The listing builds one solid part. Answer for the finished solid, in the listing's coordinates (mm). Give positions to 0.01 mm unless a question says otherwise; leave off trailing zeros. Loops run counter-clockwise (first coordinate to the right, second up) from the corner with the lowest first, then second, coordinate; pieces in that order, holes last.
Item 1: Section C-C, the plane y = -23 is taken. Give the vertices of the cut face in (x, z), and give its area (3 significant figures).
Item 2: Section B-B, the plane x = -7.5 is taken. Give the vertices of the cut face in (y, z), and give its area (3 significant figures).
Item 3: Consider line 1 along Y through (x, z) = (-45.75, 1.5); line 2 along Y through (x, z) = (11.5, 2.5); line 3 along Y through (x, z) = (-26, 7). Determine where each line is inside the solid, lowest interval first.
Item 4: Section A-A, the plane y = 45 is taken. Give the vertices of the cut face in (x, z), and give its area (4 significant figures).
Item 5: Each of these flat-tipped pins is pushed along its axis until it touches: pin 1 Ø2.5 at (x, z) = (0.5, 5.5) entering from +Y; pin 2 Ø3 at (x, y) = (38.5, -34.5) entering from +Z; pin 3 Ø4.5 at (x, z) = (-13, 5) entering from -Y. Where does it stop, or does it pass through?
from build123d import *

# Parameters (mm, degrees)
SKETCH1_W           = 100
SKETCH1_H           = 113.5
BOSS_EXTRUDE1_DEPTH = 8.5
CUT_EXTRUDE1_REACH  = 78.111
SKETCH2_W           = 83
SKETCH2_H           = 13.5
SKETCH2_H_2         = 13
SKETCH2_W_2         = 10
SKETCH2_H_3         = 10
SKETCH2_R           = 1.75
CUT_EXTRUDE2_REACH  = 78.111
SKETCH6_W           = 10
SKETCH6_H           = 10
FILLET1_R           = 1
SKETCH8_W           = 10
SKETCH8_H           = 10
CUT_EXTRUDE5_DEPTH  = 5.5
CUT_EXTRUDE6_DEPTH  = 76.834111718


with BuildPart() as part:
    # Sketch1 → Boss-Extrude1 (new body)
    with BuildSketch(Plane.XY):
        Rectangle(SKETCH1_W, SKETCH1_H)
    extrude(amount=BOSS_EXTRUDE1_DEPTH)

    # Sketch2 → Cut-Extrude1 (cut, up to next)
    with BuildSketch(Plane.XY.offset(8.5), mode=Mode.PRIVATE) as cut_extrude1_sk1:
        with Locations((0, 50)):
            Rectangle(SKETCH2_W, SKETCH2_H)
    cut_extrude1_tool1 = extrude(cut_extrude1_sk1.sketch, amount=-CUT_EXTRUDE1_REACH, mode=Mode.PRIVATE) & part.part
    # Sketch2 → Cut-Extrude1 (cut, up to next)
    with BuildSketch(Plane.XY.offset(8.5), mode=Mode.PRIVATE) as cut_extrude1_sk2:
        with BuildLine():
            ThreePointArc((-41.5, -29.75), (-39.156854249, -35.406854249), (-33.5, -37.75))
            Line((-33.5, -37.75), (33.5, -37.75))
            ThreePointArc((33.5, -37.75), (39.156854249, -35.406854249), (41.5, -29.75))
            Line((41.5, -29.75), (41.5, -0.25))
            Line((41.5, -0.25), (-41.5, -0.25))
            Line((-41.5, -0.25), (-41.5, -29.75))
        make_face()
    cut_extrude1_tool2 = extrude(cut_extrude1_sk2.sketch, amount=-CUT_EXTRUDE1_REACH, mode=Mode.PRIVATE) & part.part
    # Sketch2 → Cut-Extrude1 (cut, up to next)
    with BuildSketch(Plane.XY.offset(8.5), mode=Mode.PRIVATE) as cut_extrude1_sk3:
        with Locations((0, -50.25)):
            Rectangle(SKETCH2_W, SKETCH2_H_2)
    cut_extrude1_tool3 = extrude(cut_extrude1_sk3.sketch, amount=-CUT_EXTRUDE1_REACH, mode=Mode.PRIVATE) & part.part
    # Sketch2 → Cut-Extrude1 (cut, up to next)
    with BuildSketch(Plane.XY.offset(8.5), mode=Mode.PRIVATE) as cut_extrude1_sk4:
        with Locations((-11.75, 22.75)):
            Rectangle(SKETCH2_W_2, SKETCH2_H_3)
    cut_extrude1_tool4 = extrude(cut_extrude1_sk4.sketch, amount=-CUT_EXTRUDE1_REACH, mode=Mode.PRIVATE) & part.part
    # Sketch2 → Cut-Extrude1 (cut, up to next)
    with BuildSketch(Plane.XY.offset(8.5), mode=Mode.PRIVATE) as cut_extrude1_sk5:
        with Locations((45.75, 38.75)):
            Circle(SKETCH2_R)
    cut_extrude1_tool5 = extrude(cut_extrude1_sk5.sketch, amount=-CUT_EXTRUDE1_REACH, mode=Mode.PRIVATE) & part.part
    # Sketch2 → Cut-Extrude1 (cut, up to next)
    with BuildSketch(Plane.XY.offset(8.5), mode=Mode.PRIVATE) as cut_extrude1_sk6:
        with Locations((45.75, -38.75)):
            Circle(SKETCH2_R)
    cut_extrude1_tool6 = extrude(cut_extrude1_sk6.sketch, amount=-CUT_EXTRUDE1_REACH, mode=Mode.PRIVATE) & part.part
    # Sketch2 → Cut-Extrude1 (cut, up to next)
    with BuildSketch(Plane.XY.offset(8.5), mode=Mode.PRIVATE) as cut_extrude1_sk7:
        with Locations((-45.75, 38.75)):
            Circle(SKETCH2_R)
    cut_extrude1_tool7 = extrude(cut_extrude1_sk7.sketch, amount=-CUT_EXTRUDE1_REACH, mode=Mode.PRIVATE) & part.part
    # Sketch2 → Cut-Extrude1 (cut, up to next)
    with BuildSketch(Plane.XY.offset(8.5), mode=Mode.PRIVATE) as cut_extrude1_sk8:
        with Locations((-45.75, -38.75)):
            Circle(SKETCH2_R)
    cut_extrude1_tool8 = extrude(cut_extrude1_sk8.sketch, amount=-CUT_EXTRUDE1_REACH, mode=Mode.PRIVATE) & part.part
    add(cut_extrude1_tool1.solids().sort_by_distance((0, 50, 8.5))[0], mode=Mode.SUBTRACT)
    add(cut_extrude1_tool2.solids().sort_by_distance((0, -18.848961, 8.5))[0], mode=Mode.SUBTRACT)
    add(cut_extrude1_tool3.solids().sort_by_distance((0, -50.25, 8.5))[0], mode=Mode.SUBTRACT)
    add(cut_extrude1_tool4.solids().sort_by_distance((-11.75, 22.75, 8.5))[0], mode=Mode.SUBTRACT)
    add(cut_extrude1_tool5.solids().sort_by_distance((45.75, 38.75, 8.5))[0], mode=Mode.SUBTRACT)
    add(cut_extrude1_tool6.solids().sort_by_distance((45.75, -38.75, 8.5))[0], mode=Mode.SUBTRACT)
    add(cut_extrude1_tool7.solids().sort_by_distance((-45.75, 38.75, 8.5))[0], mode=Mode.SUBTRACT)
    add(cut_extrude1_tool8.solids().sort_by_distance((-45.75, -38.75, 8.5))[0], mode=Mode.SUBTRACT)

    # Sketch6 → Cut-Extrude2 (cut, up to next)
    with BuildSketch(Plane.XY.offset(8.5), mode=Mode.PRIVATE) as cut_extrude2_sk1:
        with BuildLine():
            Line((41.5, 8.25), (41.5, 29.25))
            ThreePointArc((41.5, 29.25), (39.156854249, 34.906854249), (33.5, 37.25))
            Line((33.5, 37.25), (28.5, 37.25))
            Line((28.5, 37.25), (28.5, 8.25))
            Line((28.5, 8.25), (33.5, 8.25))
            Line((33.5, 8.25), (41.5, 8.25))
        make_face()
    cut_extrude2_tool1 = extrude(cut_extrude2_sk1.sketch, amount=-CUT_EXTRUDE2_REACH, mode=Mode.PRIVATE) & part.part
    # Sketch6 → Cut-Extrude2 (cut, up to next)
    with BuildSketch(Plane.XY.offset(8.5), mode=Mode.PRIVATE) as cut_extrude2_sk2:
        with Locations((11.75, 22.75)):
            Rectangle(SKETCH6_W, SKETCH6_H)
    cut_extrude2_tool2 = extrude(cut_extrude2_sk2.sketch, amount=-CUT_EXTRUDE2_REACH, mode=Mode.PRIVATE) & part.part
    # Sketch6 → Cut-Extrude2 (cut, up to next)
    with BuildSketch(Plane.XY.offset(8.5), mode=Mode.PRIVATE) as cut_extrude2_sk3:
        with BuildLine():
            Line((-41.5, 8.25), (-41.5, 29.25))
            ThreePointArc((-41.5, 29.25), (-39.156854249, 34.906854249), (-33.5, 37.25))
            Line((-33.5, 37.25), (-28.5, 37.25))
            Line((-28.5, 37.25), (-28.5, 8.25))
            Line((-28.5, 8.25), (-33.5, 8.25))
            Line((-33.5, 8.25), (-41.5, 8.25))
        make_face()
    cut_extrude2_tool3 = extrude(cut_extrude2_sk3.sketch, amount=-CUT_EXTRUDE2_REACH, mode=Mode.PRIVATE) & part.part
    add(cut_extrude2_tool1.solids().sort_by_distance((34.821806, 22.269339, 8.5))[0], mode=Mode.SUBTRACT)
    add(cut_extrude2_tool2.solids().sort_by_distance((11.75, 22.75, 8.5))[0], mode=Mode.SUBTRACT)
    add(cut_extrude2_tool3.solids().sort_by_distance((-34.821806, 22.269339, 8.5))[0], mode=Mode.SUBTRACT)

    # Fillet1
    fillet1_edges = [part.edges().sort_by_distance(p)[0] for p in [
        (45.75, -56.75, 0),
        (-45.75, 56.75, 0),
        (-45.75, -56.75, 8.5),
        (-45.75, 56.75, 8.5),
        (45.75, -56.75, 8.5),
        (-41.5, 56.75, 4.25),
        (41.5, 56.75, 4.25),
        (41.5, -56.75, 4.25),
        (-41.5, -56.75, 4.25),
        (-45.75, -56.75, 0),
        (45.75, 56.75, 0),
        (50, -56.75, 4.25),
        (-50, -56.75, 4.25),
        (-50, 56.75, 4.25),
        (50, 56.75, 4.25),
        (45.75, 56.75, 8.5),
    ]]
    fillet(fillet1_edges, radius=FILLET1_R)

    # Sketch8 → Cut-Extrude5 (cut)
    with BuildSketch(Plane.XY.offset(8.5)):
        with BuildLine():
            ThreePointArc((-46.701116722, 32.72), (-46.210984272, 34.031299083), (-44.981116722, 34.7))
            ThreePointArc((-44.981116722, 34.7), (-42.571113581, 35.629410248), (-40.811116722, 37.52))
            Line((-40.811116722, 37.52), (-39.567050808, 39.7))
            ThreePointArc((-39.567050808, 39.7), (-38.836346779, 40.434383498), (-37.835, 40.7))
            Line((-37.835, 40.7), (37.835, 40.7))
            ThreePointArc((37.835, 40.7), (38.836346779, 40.434383498), (39.567050808, 39.7))
            Line((39.567050808, 39.7), (40.811116722, 37.52))
            ThreePointArc((40.811116722, 37.52), (42.571113581, 35.629410248), (44.981116722, 34.7))
            ThreePointArc((44.981116722, 34.7), (46.210984272, 34.031299083), (46.701116722, 32.72))
            Line((46.701116722, 32.72), (46.701116722, -32.72))
            ThreePointArc((46.701116722, -32.72), (46.210984272, -34.031299083), (44.981116722, -34.7))
            ThreePointArc((44.981116722, -34.7), (42.571113581, -35.629410248), (40.811116722, -37.52))
            Line((40.811116722, -37.52), (39.567050808, -39.7))
            ThreePointArc((39.567050808, -39.7), (38.836346779, -40.434383498), (37.835, -40.7))
            Line((37.835, -40.7), (-37.835, -40.7))
            Line((-37.835, -40.7), (-39.567050808, -39.7))
            Line((-39.567050808, -39.7), (-40.811116722, -37.52))
            ThreePointArc((-40.811116722, -37.52), (-42.571113581, -35.629410248), (-44.981116722, -34.7))
            ThreePointArc((-44.981116722, -34.7), (-46.210984272, -34.031299083), (-46.701116722, -32.72))
            Line((-46.701116722, -32.72), (-46.701116722, 32.72))
        make_face()
        with Locations((-11.75, 22.75)):
            Rectangle(SKETCH8_W, SKETCH8_H, mode=Mode.SUBTRACT)
        with BuildLine():
            Line((33.5, -37.75), (-33.5, -37.75))
            ThreePointArc((-33.5, -37.75), (-39.156854249, -35.406854249), (-41.5, -29.75))
            Line((-41.5, -29.75), (-41.5, -0.25))
            Line((-41.5, -0.25), (41.5, -0.25))
            Line((41.5, -0.25), (41.5, -29.75))
            ThreePointArc((41.5, -29.75), (39.156854249, -35.406854249), (33.5, -37.75))
        make_face(mode=Mode.SUBTRACT)
        with Locations((11.75, 22.75)):
            Rectangle(SKETCH8_W, SKETCH8_H, mode=Mode.SUBTRACT)
        with BuildLine():
            Line((-41.5, 8.25), (-41.5, 29.25))
            ThreePointArc((-41.5, 29.25), (-39.156854249, 34.906854249), (-33.5, 37.25))
            Line((-33.5, 37.25), (-28.5, 37.25))
            Line((-28.5, 37.25), (-28.5, 8.25))
            Line((-28.5, 8.25), (-41.5, 8.25))
        make_face(mode=Mode.SUBTRACT)
        with BuildLine():
            Line((41.5, 8.25), (28.5, 8.25))
            Line((28.5, 8.25), (28.5, 37.25))
            Line((28.5, 37.25), (33.5, 37.25))
            ThreePointArc((33.5, 37.25), (39.156854249, 34.906854249), (41.5, 29.25))
            Line((41.5, 29.25), (41.5, 8.25))
        make_face(mode=Mode.SUBTRACT)
    extrude(amount=-CUT_EXTRUDE5_DEPTH, mode=Mode.SUBTRACT)

    # Sketch9 → Cut-Extrude6 (cut, through all)
    with BuildSketch(Plane.XY.offset(3)):
        with BuildLine():
            Line((-33.5, -37.75), (33.5, -37.75))
            ThreePointArc((33.5, -37.75), (39.156854249, -35.406854249), (41.5, -29.75))
            Line((41.5, -29.75), (41.5, 29.25))
            ThreePointArc((41.5, 29.25), (39.156854249, 34.906854249), (33.5, 37.25))
            Line((33.5, 37.25), (-33.5, 37.25))
            ThreePointArc((-33.5, 37.25), (-39.156854249, 34.906854249), (-41.5, 29.25))
            Line((-41.5, 29.25), (-41.5, -29.75))
            ThreePointArc((-41.5, -29.75), (-39.156854249, -35.406854249), (-33.5, -37.75))
        make_face()
    extrude(amount=-CUT_EXTRUDE6_DEPTH, mode=Mode.SUBTRACT)


solid = part.part
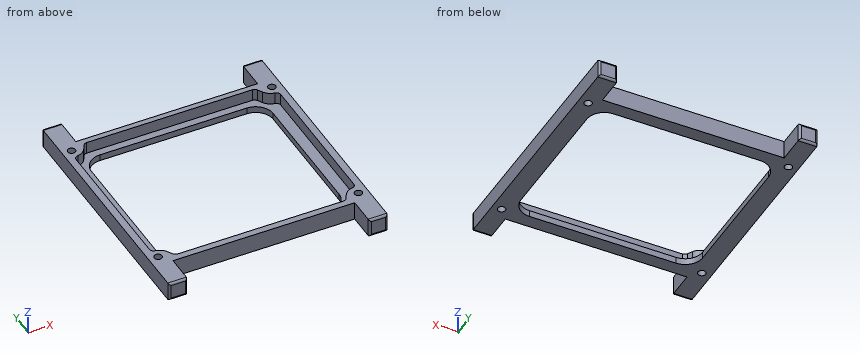
Worked answers:
1. outline: (-50, 0) - (-41.5, 0) - (-41.5, 3) - (-46.7, 3) - (-46.7, 8.5) - (-50, 8.5) - close; (41.5, 0) - (50, 0) - (50, 8.5) - (46.7, 8.5) - (46.7, 3) - (41.5, 3) - close
1. area: 87.3 mm2
2. outline: (-43.75, 0) - (-37.75, 0) - (-37.75, 3) - (-40.7, 3) - (-40.7, 8.5) - (-43.75, 8.5) - close; (37.25, 0) - (43.25, 0) - (43.25, 8.5) - (40.7, 8.5) - (40.7, 3) - (37.25, 3) - close
2. area: 66.8 mm2
3. line 1: y = -56.75 to -40.5, -37 to 37, 40.5 to 56.75
3. line 2: y = -43.75 to -37.75, 37.25 to 43.25
3. line 3: y = -43.75 to -40.7, 40.7 to 43.25
4. outline: (-50, 0) - (-41.5, 0) - (-41.5, 8.5) - (-50, 8.5) - close; (41.5, 0) - (50, 0) - (50, 8.5) - (41.5, 8.5) - close
4. area: 144.5 mm2
5. pin 1: stops at y = 43.25
5. pin 2: stops at z = 3
5. pin 3: stops at y = -43.75
